Geometry: see drawing. Coordinates: mm, zero at the bounding-box minimum. A direction names the side the tool comes from. Give positions to 0.01 mm unless a question says otherwise; leave off trailing zeros. Loops run counter-clockwise (first coordinate to the right, second up) from the corner with the lowest first, then second, coordinate; pieces in that order, holes last. Notation, with made-up numbers: M -23.75,30 L 21.25,30 A29 ccw 21.25,64 Z; hole C 66.5,59.25 d2. An arc over 180 degrees is marked long. Put each result on its own line as item: value.
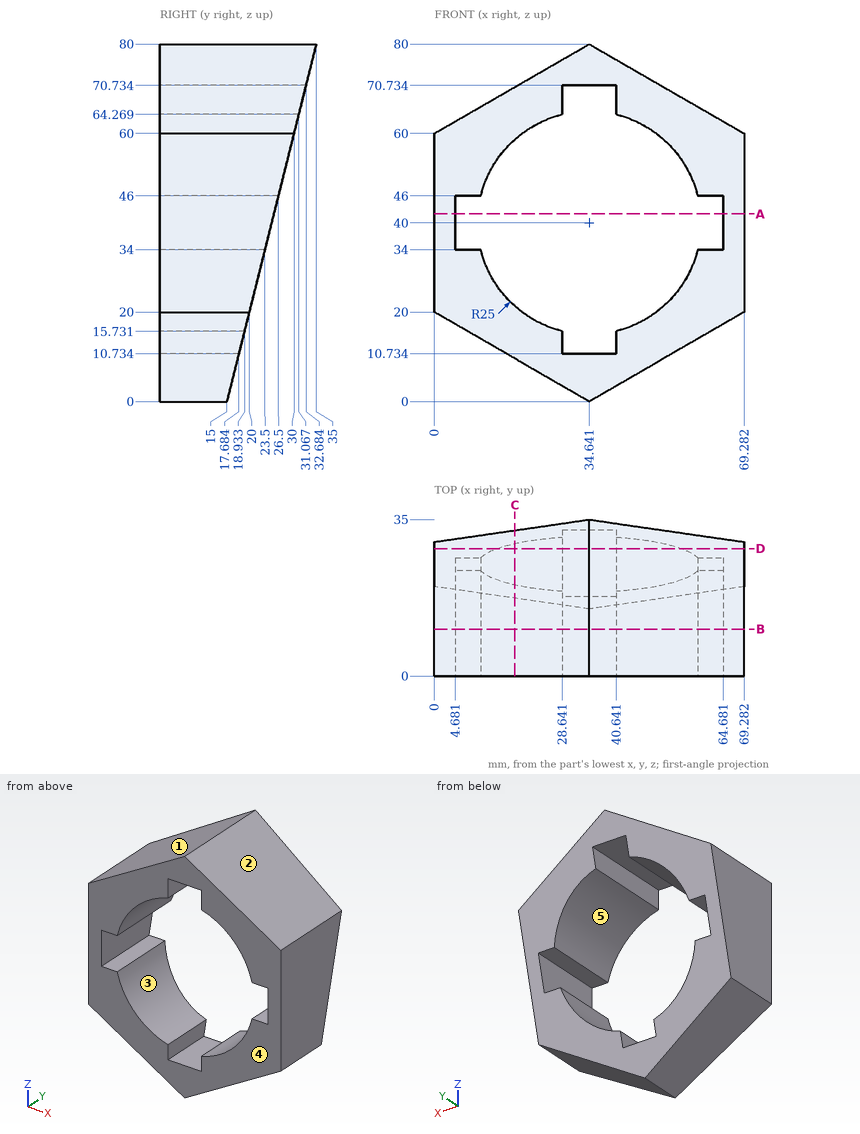
Item 1: Section A-A on z = 42. Output: boundary loops of the cut face in (x, y).
Output values:
outline: M 0,0 L 4.68,0 L 4.68,25.5 L 0,25.5 Z; M 64.68,0 L 69.28,0 L 69.28,25.5 L 64.68,25.5 Z
Item 2: Section B-B on y = 10.5. Output: boundary loops of the cut face in (x, z) (1 decimal), then the cut area to 3 significant figures.
Output values:
outline: M 0,20 L 34.6,0 L 69.3,20 L 69.3,60 L 34.6,80 L 0,60 Z; hole M 4.7,34 L 10.4,34 A25 ccw 28.6,15.7 L 28.6,10.7 L 40.6,10.7 L 40.6,15.7 A25 ccw 58.9,34 L 64.7,34 L 64.7,46 L 58.9,46 A25 ccw 40.6,64.3 L 40.6,70.7 L 28.6,70.7 L 28.6,64.3 A25 ccw 10.4,46 L 4.7,46 Z
area: 1,940 mm²
Item 3: Set-up query: the marked faces 4 and 5. Return all of +Z, -Z, +X, -X, +Y, -Y with unobstructed straight access to the full face (end or side cutting, diameter ignored); none if empty.
Output values:
face 4: +Z, -Z, +X, -X, -Y
face 5: +Y, -Y
Item 4: Line query: probe 1 along X at (y, z) = (12, 41); probe 2 along Z at (x, y) = (56.5, 4) (1 decimal); probe 3 along Z at (x, y) = (64.5, 1). Output: solid intervals per line, ascending. Write a range as [from, to].
Output values:
probe 1: [0, 4.68], [64.68, 69.28]
probe 2: [12.6, 27.9], [52.1, 67.4]
probe 3: [17.24, 34], [46, 62.76]
Item 5: Mould query, pull axis X, two halves, no side actions, for the marked faces 1, 2 and 3. Classes: pulls with the +X half, pulls with the -X half, needs draft (parallel to the pull), parting line crosses it, or undercut.
Output values:
face 1: pulls with the -X half
face 2: pulls with the +X half
face 3: undercut
Item 6: Pin query (flat end, axial travel): pin 1 Ø1.5 at (y, z) = (12, 14) entering from -X (1 decimal); pin 2 Ø4.5 at (x, y) = (8, 15.5) entering from +Z; pin 3 Ø6.5 at (x, y) = (61.5, 19.5) entering from -Z (1 decimal); pin 4 Ø3 at (x, z) = (13.5, 46.5) entering from +Y. Return the tip coordinate at first contact, or that it passes through.
Output values:
pin 1: x = 9.1
pin 2: z = 65.92
pin 3: z = 13.7
pin 4: through
Item 7: Section C-C on x = 18. Output: boundary loops of the cut face in (y, z) (1 decimal).
Output values:
outline: M 0,9.6 L 17.4,9.6 L 20.3,21.3 L 0,21.3 Z; M 0,58.7 L 29.7,58.7 L 32.6,70.4 L 0,70.4 Z
Item 8: Section D-D on y = 28.5. Output: boundary loops of the cut face in (x, z) (1 decimal).
Output values:
outline: M 0,54 L 13.9,54 A25 cw 28.6,64.3 L 28.6,70.7 L 40.6,70.7 L 40.6,64.3 A25 cw 55.4,54 L 69.3,54 L 69.3,60 L 34.6,80 L 0,60 Z
